from build123d import *

# Parameters (mm, degrees)
F0_R     = 1.65
F2_DEPTH = 90
F1_W     = 60
F1_H     = 5
F3_DEPTH = 42
F4_DEPTH = 97


with BuildPart() as f2:
    # F0 (on Top) → F2 (new body)
    with BuildSketch(Plane.XY):
        Polygon((-49.989993, -7.976015), (10.010007, -7.976015), (10.010007, 2.023985), (-49.989994, 2.023985), align=None)
        with Locations((-44.239994, -2.976015)):
            Circle(F0_R, mode=Mode.SUBTRACT)
        with Locations((4.240008, -2.976015)):
            Circle(F0_R, mode=Mode.SUBTRACT)
    extrude(amount=F2_DEPTH)

    # F1 (on Front) → F3 (join)
    with BuildSketch(Plane.XZ):
        with Locations((-20.000001, 87.5)):
            Rectangle(F1_W, F1_H)
    extrude(amount=-F3_DEPTH)

    # F0 (on Top) → F4 (cut)
    with BuildSketch(Plane.XY):
        with Locations((4.240008, -2.976015)):
            Circle(F0_R)
        with Locations((-44.239994, -2.976015)):
            Circle(F0_R)
        with Locations((-38.499993, 34.023985)):
            Circle(F0_R)
        with Locations((-1.499993, 34.023985)):
            Circle(F0_R)
    extrude(amount=F4_DEPTH, mode=Mode.SUBTRACT)


solid = f2.part
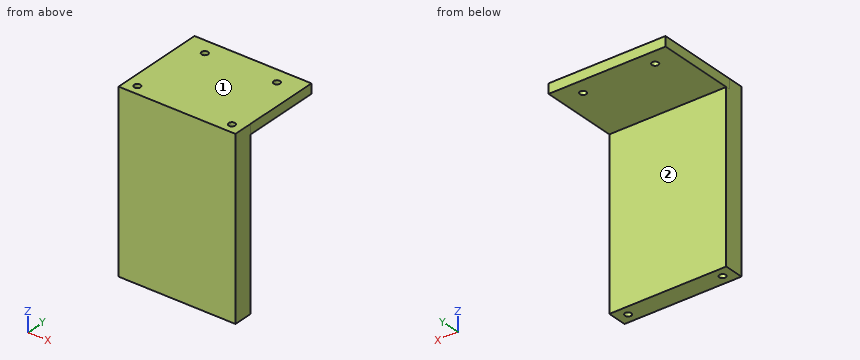
Geometry check sheet. Reference: the model listing, model coordinates, mm. Face numbers are marked on the shaded views. A direction names the side the tool comes from. Give positions to 0.01 mm unless a question says otherwise; leave off trailing zeros. Write each loop counter-clockwise with the first axis right and the second up, starting at its lowest first coordinate (ties: lowest second). Pieces come first, ordered by that corner, then holes. Notation, with made-up numbers: (-22.75, 11.5) - (-9.75, 11.5) arc R19 cw to (-9.75, 21.5) - close; hole circle Ø1 at (48.5, 5.25). An arc over 180 degrees is marked (long way). Put each result on its own line as item: value.
1. Sectioned sample at D-D, the plane y = 18.5. Enter the section's corners in (x, z), plus the area to 3 significant figures.
Ans:
outline: (-50, 85) - (10, 85) - (10, 90) - (-50, 90) - close
area: 300 mm²
2. Sectioned sample at C-C, the plane x = -34. Enter the section's corners in (y, z), plus the area to 3 significant figures.
Ans:
outline: (-7.98, 0) - (2.02, 0) - (2.02, 85) - (42, 85) - (42, 90) - (-7.98, 90) - close
area: 1,100 mm²
3. Go/stop test with flat-tipped pins: pin 1 (12.5 mm diameter, centred on x = -29, y = 14.5, fed in from -Z); pin 2 (4 mm diameter, centred on x = -33.5, z = 30, fed in from +Y); pin 3 (5.5 mm diameter, centred on y = 19.5, z = 87.5, fed in from +X); pin 4 (2.5 mm diameter, centred on x = -1.5, y = 34.02, fed in from +Z). Record where each tip stops, or that it passes through.
Ans:
pin 1: stops at z = 85
pin 2: stops at y = 2.02
pin 3: stops at x = 10
pin 4: passes through
4. Thickness scan on line 1 (X direction, y = -4, z = 59.5); line 2 (Z direction, x = -30.5, y = 4.5); line 3 (Y direction, x = -39, z = 47.5). Record the ranges inside material, lowest first.
Ans:
line 1: x = -49.99 to -45.53, -42.95 to 2.95, 5.53 to 10.01
line 2: z = 85 to 90
line 3: y = -7.98 to 2.02
5. Set-up check for the marked faces 1 and 2: record each of +Z, -Z, +X, -X, +Y, -Y from which the full face is reachable in a straight line by a thin tool's end or side.
Ans:
face 1: +Z, +X, -X, +Y, -Y
face 2: -Z, +X, -X, +Y
6. Sectioned sample at A-A, the plane x = -44. Enter the section's corners in (y, z), plus the area to 3 significant figures.
Ans:
outline: (-7.98, 0) - (-4.61, 0) - (-4.61, 90) - (-7.98, 90) - close; (-1.34, 0) - (2.02, 0) - (2.02, 85) - (42, 85) - (42, 90) - (-1.34, 90) - close
area: 806 mm²
7. Sectioned sample at B-B, the plane z = 26.5. Enter the section's corners in (x, y).
Ans:
outline: (-49.99, -7.98) - (10.01, -7.98) - (10.01, 2.02) - (-49.99, 2.02) - close; hole circle Ø3.3 at (-44.24, -2.98); hole circle Ø3.3 at (4.24, -2.98)
